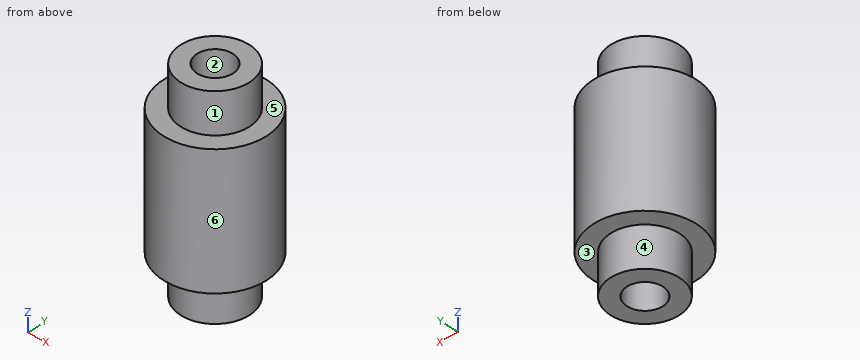
Autodesk Inventor part; units mm, degrees
ref_plane "Work Plane1" through (0, 0, 6.35) normal (0, 0, 1) x (1, 0, 0)
ref_plane "YZ Plane" through (0, 0, 0) normal (1, 0, 0) x (0, 1, 0)
ref_plane "XZ Plane" through (0, 0, 0) normal (0, 1, 0) x (-1, 0, 0)
sketch "Sketch1" plane through (0, 0, 0) normal (0, 0, 1) x (1, 0, 0)
  circle A0 centre (0, 0) radius 7.1437
  dimension "d0" = 14.2875
extrude "Extrusion1" add sketch "Sketch1" along normal blind 18.0975
ref_plane "Work Plane1" through (0, 0, 6.35) normal (0, 0, 1) x (1, 0, 0)
sketch "Sketch6" plane through (0, 0, 18.0975) normal (0, 0, 1) x (1, 0, 0)
  circle A0 centre (0, 0) radius 2.4892
  dimension "d28" = 4.9784
extrude "Extrusion3" cut sketch "Sketch6" against normal through all
sketch "Sketch7" plane through (0, 0, 18.0975) normal (0, 0, 1) x (1, 0, 0)
  circle A0 centre (0, 0) radius 4.7625
  circle A1 centre (0, 0) radius 2.4892
  dimension "d31" = 9.525
  dimension "d32" = 4.9784
extrude "Extrusion4" add sketch "Sketch7" along normal blind 5.5563
sketch "Sketch8" plane through (0, 0, 0) normal (0, 0, -1) x (-1, 0, 0)
  circle A0 centre (0, 0) radius 2.4892
  circle A1 centre (0, 0) radius 4.7625
extrude "Extrusion5" add sketch "Sketch8" along normal blind 5.5563
properties part number "RollerSpacer2(Bearing)"
Input: part model. Units: mm. Frame: model coordinates. Face numbers are marked on the shaded views. A direction names the side the tool comes from. Coordinates: 2 decimals unless noted, no trailing zeros. Loops run counter-clockwise (first coordinate to the right, second up) from the corner with the lowest first, then second, coordinate; pieces in that order, holes last.
Q1. Draft query along X for the marked faces 1, 2 and 3. Return one class per face: +X half, -X half, draft (parallel to the pull), parting line (faces both ways), or undercut.
Q2. Cut plane D-D (y = 3). Output: boundary loops of the cut face in (x, z).
Q3. Cut plane A-A (y = 0). Output: boundary loops of the cut face in (x, z), then the cut area to 3 significant figures.
Q4. Contact query for flat-ended pins moving along their axis: pin 1 (6 mm diameter, centred on x = -2, y = -5, fed in from -Z); pin 2 (6 mm diameter, centred on y = 5.5, z = 6, fed in from -X); pin 3 (5 mm diameter, centred on x = -5.5, z = 6, fed in from +Y); pin 4 (8 mm diameter, centred on x = -5, z = 16.5, fed in from -Y). Output: stop coordinate, or through.
Q5. Set-up query: the marked faces 4, 5 and 6. Return all of +Z, -Z, +X, -X, +Y, -Y with unobstructed straight access to the full face (end or side cutting, diameter ignored); none if empty.
Q6. Material intervals for line 1 (Y direction, x = 0, z = 8.5); line 2 (Z direction, x = -4.5, y = -2.5); line 3 (X direction, y = 0.75, z = -0.25), sorted ascending.
Q7. Cut plane C-C (z = 20.5). Output: boundary loops of the cut face in (x, y) (1 decimal).
Working result:
1. face 1: parting line
1. face 2: undercut
1. face 3: draft
2. outline: (-6.48, 0) - (-3.7, 0) - (-3.7, -5.56) - (3.7, -5.56) - (3.7, 0) - (6.48, 0) - (6.48, 18.1) - (3.7, 18.1) - (3.7, 23.65) - (-3.7, 23.65) - (-3.7, 18.1) - (-6.48, 18.1) - close
3. outline: (-7.14, 0) - (-4.76, 0) - (-4.76, -5.56) - (-2.49, -5.56) - (-2.49, 23.65) - (-4.76, 23.65) - (-4.76, 18.1) - (-7.14, 18.1) - close; (2.49, -5.56) - (4.76, -5.56) - (4.76, 0) - (7.14, 0) - (7.14, 18.1) - (4.76, 18.1) - (4.76, 23.65) - (2.49, 23.65) - close
3. area: 219 mm2
4. pin 1: stops at z = -5.56
4. pin 2: stops at x = -6.69
4. pin 3: stops at y = 6.48
4. pin 4: stops at y = -7.07
5. face 4: -Z
5. face 5: +Z
5. face 6: +Z, -Z
6. line 1: y = -7.14 to -2.49, 2.49 to 7.14
6. line 2: z = 0 to 18.1
6. line 3: x = -4.7 to -2.37, 2.37 to 4.7
7. outline: circle Ø9.5 at (0, 0); hole circle Ø5 at (0, 0)
